from build123d import *

# Parameters (mm, degrees)
SKETCH2_R           = 76
BOSS_EXTRUDE1_DEPTH = 17.78
CUT_EXTRUDE3_DEPTH  = 13.97
CUT_EXTRUDE5_DEPTH  = 1.27
SKETCH10_W          = 41.91
SKETCH10_H          = 10.16
CUT_EXTRUDE6_DEPTH  = 1.016
SKETCH11_W          = 44.45
SKETCH11_H          = 44.45
BOSS_EXTRUDE2_DEPTH = 1.27
SKETCH14_R          = 3.175
BOSS_EXTRUDE4_DEPTH = 5.08
SKETCH15_R          = 73.66
BOSS_EXTRUDE5_DEPTH = 2.54


with BuildPart() as part:
    # Sketch2 → Boss-Extrude1 (new body)
    with BuildSketch(Plane(origin=(0, 0, 0), x_dir=(1, 0, 0), z_dir=(0, 1, 0))):
        Circle(SKETCH2_R)
    extrude(amount=BOSS_EXTRUDE1_DEPTH)

    # Sketch6 → Cut-Extrude3 (cut)
    with BuildSketch(Plane(origin=(0, 17.78, 0), x_dir=(1, 0, 0), z_dir=(0, 1, 0))):
        with BuildLine():
            Line((-76, 54.61), (76, 54.61))
            ThreePointArc((76, 54.61), (130.61, 0), (76, -54.61))
            Line((76, -54.61), (-76, -54.61))
            ThreePointArc((-76, -54.61), (-130.61, 0), (-76, 54.61))
        make_face()
    extrude(amount=-CUT_EXTRUDE3_DEPTH, mode=Mode.SUBTRACT)

    # Sketch9 → Cut-Extrude5 (cut)
    with BuildSketch(Plane(origin=(0, 3.81, 0), x_dir=(1, 0, 0), z_dir=(0, 1, 0))):
        with BuildLine():
            Line((-76, 25.4), (-25.4, 25.4))
            Line((-25.4, 25.4), (25.4, 25.4))
            Line((25.4, 25.4), (76, 25.4))
            ThreePointArc((76, 25.4), (101.4, 0), (76, -25.4))
            Line((76, -25.4), (25.4, -25.4))
            Line((25.4, -25.4), (-25.4, -25.4))
            Line((-25.4, -25.4), (-76, -25.4))
            ThreePointArc((-76, -25.4), (-101.4, 0), (-76, 25.4))
        make_face()
    extrude(amount=-CUT_EXTRUDE5_DEPTH, mode=Mode.SUBTRACT)

    # Sketch10 → Cut-Extrude6 (cut)
    with BuildSketch(Plane(origin=(0, 2.54, 0), x_dir=(1, 0, 0), z_dir=(0, 1, 0))):
        with Locations((-48.79885899, 13.97)):
            Rectangle(SKETCH10_W, SKETCH10_H)
        with Locations((-48.79885899, -13.97)):
            Rectangle(SKETCH10_W, SKETCH10_H)
        with Locations((48.79885899, -13.97)):
            Rectangle(SKETCH10_W, SKETCH10_H)
        with Locations((48.79885899, 13.97)):
            Rectangle(SKETCH10_W, SKETCH10_H)
    extrude(amount=-CUT_EXTRUDE6_DEPTH, mode=Mode.SUBTRACT)

    # Sketch11 → Boss-Extrude2 (add)
    with BuildSketch(Plane(origin=(0, 2.54, 0), x_dir=(1, 0, 0), z_dir=(0, 1, 0))):
        Rectangle(SKETCH11_W, SKETCH11_H)
    extrude(amount=BOSS_EXTRUDE2_DEPTH)

    # Sketch14 → Boss-Extrude4 (add)
    with BuildSketch(Plane(origin=(0, 3.81, 0), x_dir=(1, 0, 0), z_dir=(0, 1, 0))):
        Circle(SKETCH14_R)
    extrude(amount=BOSS_EXTRUDE4_DEPTH)

    # Sketch15 → Boss-Extrude5 (add)
    with BuildSketch(Plane.XZ):
        Circle(SKETCH15_R)
    extrude(amount=BOSS_EXTRUDE5_DEPTH)


solid = part.part
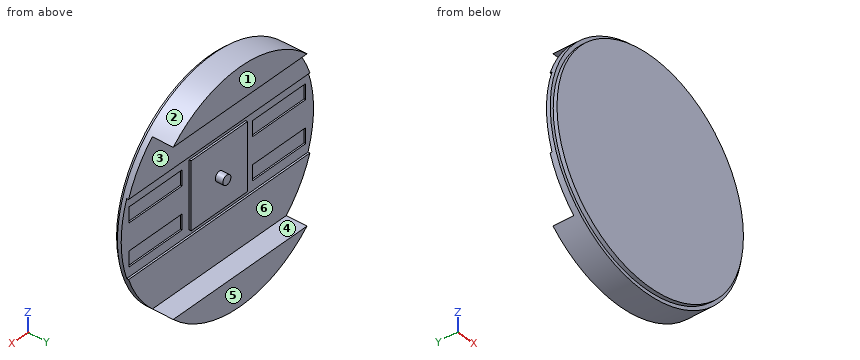
Could you check a few things on this model? Use its own coordinates, in mm. Face numbers are marked on the shaded views. A direction names the side the tool comes from. Coordinates: 2 decimals unless noted, no trailing zeros. Write each loop counter-clockwise with the first axis right and the second up, starting at its lowest first coordinate (ties: lowest second). Pieces come first, ordered by that corner, then holes. Notation, with made-up numbers: (89, -4.5) - (112, -4.5) arc R26 ccw to (112, 28.5) - close; hole circle Ø4 at (16, -17.5). An arc over 180 degrees is marked (long way). Put each result on its own line as item: value. Start each with the question number.
Q1. Thinking about a two-plate mould opening in Z: for the marked faces 1, 2, 3 and 4, which applies, pulls with the +Z half, pulls with the -Z half, needs draft (parallel to the pull), parting line crosses it, or undercut?
Q2. I want a section at B-B on y = 13.5. Write out the boundary of the cut face in (x, z), plus the area to 3 significant figures.
Q3. I want a section at C-C on z = 0. Write out the boundary of the cut face in (x, y) (3 decimals), plus the area to 3 significant figures.
Q4. Please list where these lines run through material, in increasing order: L1, parallel to Y at x = -11, z = 54.5; L2, parallel to Z at x = -45.5, y = 7.5; L3, parallel to Z at x = 12.5, y = 16.5 (3 decimals).
Q5. I want a section at A-A on x = 0. Write out the boundary of the cut face in (y, z) (3 decimals), plus the area to 3 significant figures.
Q6. I want a section at D-D on x = 62.5. Write out the boundary of the cut face in (y, z).
Q7. Which directions (+Z, -Z, +X, -X, +Y, -Y) give clear straight access to the entire face, cutting with the end or side of a thin tool? Please do the marked faces 5 and 6.
Q8. I'm going to push flat-ended pins straight in: P1, Ø6, axis at x = -57, z = 39, coming from the +Y side; P2, Ø0.6, axis at x = -7, y = 3.5, coming from the +Z side; P3, Ø10, axis at y = 13.5, z = 3, coming from the +X side. Where does each tip first touch, or does it pass through?
Checks:
1. face 1: needs draft
1. face 2: parting line crosses it
1. face 3: undercut
1. face 4: undercut
2. outline: (-52.86, -54.61) arc R76 ccw to (52.86, -54.61) - close; (-52.86, 54.61) - (52.86, 54.61) arc R76 ccw to start
2. area: 3,110 mm²
3. outline: (-76, 0) - (-73.66, 0) - (-73.66, -2.54) - (73.66, -2.54) - (73.66, 0) - (76, 0) - (76, 2.54) - (22.225, 2.54) - (22.225, 3.81) - (3.175, 3.81) - (3.175, 8.89) - (-3.175, 8.89) - (-3.175, 3.81) - (-22.225, 3.81) - (-22.225, 2.54) - (-76, 2.54) - close
3. area: 849 mm²
4. L1: -2.54 to 3.81
4. L2: -60.87 to -54.61, 54.61 to 60.87
4. L3: -74.965 to -54.61, 54.61 to 74.965
5. outline: (-2.54, -73.66) - (0, -73.66) - (0, -76) - (17.78, -76) - (17.78, -54.61) - (3.81, -54.61) - (3.81, -25.4) - (2.54, -25.4) - (2.54, -22.225) - (3.81, -22.225) - (3.81, -3.175) - (8.89, -3.175) - (8.89, 3.175) - (3.81, 3.175) - (3.81, 22.225) - (2.54, 22.225) - (2.54, 25.4) - (3.81, 25.4) - (3.81, 54.61) - (17.78, 54.61) - (17.78, 76) - (0, 76) - (0, 73.66) - (-2.54, 73.66) - close
5. area: 1,580 mm²
6. outline: (-2.54, -38.98) - (0, -38.98) - (0, -43.24) - (3.81, -43.24) - (3.81, -25.4) - (2.54, -25.4) - (2.54, -19.05) - (1.52, -19.05) - (1.52, -8.89) - (2.54, -8.89) - (2.54, 8.89) - (1.52, 8.89) - (1.52, 19.05) - (2.54, 19.05) - (2.54, 25.4) - (3.81, 25.4) - (3.81, 43.24) - (0, 43.24) - (0, 38.98) - (-2.54, 38.98) - close
7. face 5: +Z, -Z, +X, -X, +Y
7. face 6: +X, -X, +Y
8. P1: y = 3.81
8. P2: z = 75.7
8. P3: x = 2.99
